from build123d import *

# Parameters (mm, degrees)
SKETCH1_W           = 95
SKETCH1_H           = 38
BOSS_EXTRUDE1_DEPTH = 6
SKETCH2_W           = 95
SKETCH2_H           = 38
BOSS_EXTRUDE2_DEPTH = 6
SKETCH11_W          = 20.001105266
SKETCH11_H          = 64
BOSS_EXTRUDE5_DEPTH = 6
SKETCH13_W          = 10
SKETCH13_H          = 9
BOSS_EXTRUDE7_DEPTH = 6
SKETCH16_R          = 9
CUT_EXTRUDE2_DEPTH  = 6
SKETCH20_R          = 13.05
CUT_EXTRUDE3_DEPTH  = 5
CUT_EXTRUDE4_START  = -6
SKETCH21_R          = 8
SKETCH21_R_2        = 9
CUT_EXTRUDE4_DEPTH  = 6
CUT_EXTRUDE5_START  = -5
SKETCH22_R          = 13.05
CUT_EXTRUDE5_DEPTH  = 5
SKETCH25_R          = 2.5
CUT_EXTRUDE6_DEPTH  = 6
FILLET2_R           = 6


with BuildPart() as part:
    # Sketch1 → Boss-Extrude1 (new body)
    with BuildSketch(Plane.XY):
        with Locations((7.938087136, 9.487020953)):
            Rectangle(SKETCH1_W, SKETCH1_H)
    extrude(amount=BOSS_EXTRUDE1_DEPTH)



with BuildPart() as body_2:
    # Sketch2 → Boss-Extrude2 (new body)
    with BuildSketch(Plane.XY.offset(70)):
        with Locations((7.938087136, 9.487020953)):
            Rectangle(SKETCH2_W, SKETCH2_H)
    extrude(amount=BOSS_EXTRUDE2_DEPTH)


with BuildPart() as part_1:
    add(part.part)

    add(body_2.part)  # Boss-Extrude5 merges body 2
    # Sketch11 → Boss-Extrude5 (add)
    with BuildSketch(Plane(origin=(0, -9.512979047, 0), x_dir=(-1, 0, 0), z_dir=(0, -1, 0))):
        with Locations((-45.437534503, -38)):
            Rectangle(SKETCH11_W, SKETCH11_H)
    extrude(amount=-BOSS_EXTRUDE5_DEPTH)

    # Sketch13 → Boss-Extrude7 (add)
    with BuildSketch(Plane(origin=(0, -9.512979047, 0), x_dir=(-1, 0, 0), z_dir=(0, -1, 0))):
        with Locations((34.561912864, -65.5)):
            Rectangle(SKETCH13_W, SKETCH13_H)
    extrude(amount=-BOSS_EXTRUDE7_DEPTH)

    # Sketch16 → Cut-Extrude2 (cut)
    with BuildSketch(Plane.XY.offset(76)):
        with Locations((-24.561912864, 7.987020953)):
            Circle(SKETCH16_R)
        with Locations((8.438087136, 7.987020953)):
            Circle(SKETCH16_R)
    extrude(amount=-CUT_EXTRUDE2_DEPTH, mode=Mode.SUBTRACT)

    # Sketch20 → Cut-Extrude3 (cut)
    with BuildSketch(Plane.XY.offset(76)):
        with Locations((-24.561912864, 7.987020953)):
            Circle(SKETCH20_R)
        with Locations((8.438087136, 7.987020953)):
            Circle(SKETCH20_R)
    extrude(amount=-CUT_EXTRUDE3_DEPTH, mode=Mode.SUBTRACT)

    # Sketch21 → Cut-Extrude4 (cut)
    with BuildSketch(Plane(origin=(0, 0, 0), x_dir=(-1, 0, 0), z_dir=(0, 0, -1)).offset(CUT_EXTRUDE4_START)):
        with Locations((24.561912864, 7.987020953)):
            Circle(SKETCH21_R)
        with Locations(Location((-8.438087136, 7.987020953, 0), (0, 0, 180))):
            Circle(SKETCH21_R_2)
    extrude(amount=CUT_EXTRUDE4_DEPTH, mode=Mode.SUBTRACT)

    # Sketch22 → Cut-Extrude5 (cut)
    with BuildSketch(Plane(origin=(0, 0, 0), x_dir=(-1, 0, 0), z_dir=(0, 0, -1)).offset(CUT_EXTRUDE5_START)):
        with Locations(Location((-8.438087136, 7.987020953, 0), (0, 0, 180))):
            Circle(SKETCH22_R)
    extrude(amount=CUT_EXTRUDE5_DEPTH, mode=Mode.SUBTRACT)

    # Sketch25 → Cut-Extrude6 (cut)
    with BuildSketch(Plane(origin=(0, -3.512979047, 0), x_dir=(1, 0, 0), z_dir=(0, 1, 0))):
        with Locations(Location((45.437534503, -10, 0), (0, 0, 270))):
            Circle(SKETCH25_R)
        with Locations(Location((45.437534503, -66, 0), (0, 0, 270))):
            Circle(SKETCH25_R)
        with Locations(Location((-34.561912864, -66, 0), (0, 0, 270))):
            Circle(SKETCH25_R)
    extrude(amount=-CUT_EXTRUDE6_DEPTH, mode=Mode.SUBTRACT)

    # Fillet2
    fillet2_edges = [part_1.edges().sort_by_distance(p)[0] for p in [
        (35.43698187, -6.512979047, 6),
        (35.43698187, -6.512979047, 70),
        (-29.561912864, -6.512979047, 70),
    ]]
    fillet(fillet2_edges, radius=FILLET2_R)


solid = part_1.part
Could you check a few things on this model? Use its own coordinates, in mm. A direction names the side the tool comes from. Coordinates: 2 decimals unless noted, no trailing zeros. Loops run counter-clockwise (first coordinate to the right, second up) from the corner with the lowest first, then second, coordinate; pieces in that order, holes last.
1. For faces 1 (the face through (-19.724, 15.576, 70.507)), 2 (the face through (33.726, -6.471, 7.804)), 3 (the face through (-27.851, -6.471, 68.196)), 4 (the face through (46, -3.513, 38)), 5 (the face through (5, 17, 5)), which set-ups out of +Z, -Z, +X, -X, +Y, -Y let a thin tool reach every point of the face, with its end or its side?
2. I need wall thicknesses on L1, parallel to Z at x = -12.5, y = 23; L2, parallel to X at y = -4.85, z = 66; L3, parallel to Z at x = -14, y = 9.5. Which ranges of each line are inside material? Lowest first, please.
3. Imagine slicing it at B-B (x = 39). Please give me the cut outline in (y, z).
4. Imagine slicing it at C-C (z = 66). Please give me the cut outline in (x, y).
5. We'd pull the mould along Z, two halves only. Please class faces 6 (the face through (33.63, -6.47, 68.29)), 7 (the face through (-18.54, -3.59, 73.54)), 8 (the face through (-29.562, -7, 63)), 9 (the face through (-28, -1, 71)): released by +Z, released by -Z, zero draft, split by the parting line, or undercut.
6. Imagine slicing it at D-D (z = 10). Please give me the cut outline in (x, y), and give its area (3 significant figures).
7. Imagine slicing it at A-A (y = 25). Please give me the cut outline in (x, z), and give its area (3 significant figures).
8. For P1, Ø13, axis at x = 3.5, y = 7, coming from the +Z side, with a flat end and sliding along its axis, tell me the tip position at first contact or that it passes through.
Computed values:
1. face 1: +Z
1. face 2: -X, +Y, -Y
1. face 3: +Y, -Y
1. face 4: +X, -X, +Y
1. face 5: -Z
2. L1: z = 0 to 6, 70 to 76
2. L2: x = -39.56 to -37.06, -32.06 to -29.22, 35.09 to 42.94, 47.94 to 55.44
2. L3: z = 0 to 6, 70 to 71
3. outline: (-9.51, 0) - (28.49, 0) - (28.49, 6) - (-3.51, 6) - (-3.51, 70) - (28.49, 70) - (28.49, 76) - (-9.51, 76) - close
4. outline: (-39.56, -9.51) - (-37.06, -9.51) - (-37.06, -3.51) - (-39.56, -3.51) - close; (-32.06, -9.51) - (-29.22, -9.51) - (-29.22, -3.51) - (-32.06, -3.51) - close; (35.09, -9.51) - (42.94, -9.51) - (42.94, -3.51) - (35.09, -3.51) - close; (47.94, -9.51) - (55.44, -9.51) - (55.44, -3.51) - (47.94, -3.51) - close
5. face 6: undercut
5. face 7: zero draft
5. face 8: undercut
5. face 9: released by +Z
6. outline: (35.09, -9.51) - (42.94, -9.51) - (42.94, -3.51) - (35.09, -3.51) - close; (47.94, -9.51) - (55.44, -9.51) - (55.44, -3.51) - (47.94, -3.51) - close
6. area: 92.1 mm2
7. outline: (-39.56, 0) - (55.44, 0) - (55.44, 6) - (-39.56, 6) - close; (-39.56, 70) - (55.44, 70) - (55.44, 76) - (-39.56, 76) - close
7. area: 1,140 mm2
8. P1: stops at z = 71
